Read the model definition and answer for the solid it produces. Units are mm, in the model's axes. Coordinates: 2 decimals unless noted, no trailing zeros. Order: outer loops, then holes, each group sorted by start corner. A loop starts at its lowest first (then second) coordinate and runs counter-clockwise, first axis right, second up. Notation, with made-up numbers: M 24,25.5 L 37,25.5 A17 cw 37,29.5 Z; hole C 51.5,64 d8. An arc over 180 degrees is marked long. Write each question's results on one line, items separated by ' | '.
Autodesk Inventor part; units mm, degrees
ref_plane "YZ Plane" through (0, 0, 0) normal (1, 0, 0) x (0, 1, 0)
ref_plane "XZ Plane" through (0, 0, 0) normal (0, 1, 0) x (-1, 0, 0)
ref_plane "XY Plane" through (0, 0, 0) normal (0, 0, 1) x (1, 0, 0)
sketch "Sketch1" plane through (0, 0, 0) normal (0, 1, 0) x (-1, 0, 0)
  line L0 (9.5, 3) -> (-9.5, 3)
  line L1 (-9.5, -3) -> (9.5, -3)
  circle A0 centre (-9.5, 0) radius 3
  circle A1 centre (9.5, 0) radius 3
  circle A2 centre (-9.5, 0) radius 0.05
  circle A3 centre (9.5, 0) radius 0.05
  line L2 (-9.5, 3) -> (9.5, 3)
  line L3 (-9.5, -3) -> (9.5, -3)
  arc A4 (-9.5, 3) -> (-9.5, -3) centre (-9.5, 0) ccw
  arc A5 (9.5, -3) -> (9.5, 3) centre (9.5, 0) ccw
  point P0 (0, 0)
  dimension "d0" = 19
  dimension "d1" = 6
  dimension "d2" = 0.1
  dimension "d3" = 0.1
extrude "Extrusion1" add sketch "Sketch1" along normal blind 2
properties part number "tahlo_sablona_servo"
(1) Straight lines are drawn through the part: line 1 (X direction, y = 1.15, z = -0.1); line 2 (X direction, y = 0.85, z = 1.85); line 3 (Z direction, x = -11.25, y = 0.2). For each, find the intervals that lie inside material, in ascending order.
Conclusion:
line 1: -12.5 to 12.5 | line 2: -11.86 to 11.86 | line 3: -2.44 to 2.44
(2) The part is cut by section C-C, the plane z = -1.45. Write down the section's boundary in (x, y).
Conclusion:
outline: M -12.13,0 L 12.13,0 L 12.13,2 L -12.13,2 Z
(3) The part is cut by section A-A, the plane y = 1.35. Write down the section's boundary in (x, z), then the cut area to 3 significant figures.
Conclusion:
outline: M -9.5,-3 L 9.5,-3 A3 ccw 9.5,3 L -9.5,3 A3 ccw Z; hole C -9.5,0 d0.1; hole C 9.5,0 d0.1 | area: 142 mm²
(4) The part is cut by section B-B, the plane z = -2.5. Write down the section's boundary in (x, y).
Conclusion:
outline: M -11.16,0 L 11.16,0 L 11.16,2 L -11.16,2 Z
